Autodesk Inventor part; units mm, degrees
ref_plane "YZ Plane" through (0, 0, 0) normal (1, 0, 0) x (0, 1, 0)
ref_plane "XZ Plane" through (0, 0, 0) normal (0, 1, 0) x (-1, 0, 0)
ref_plane "XY Plane" through (0, 0, 0) normal (0, 0, 1) x (1, 0, 0)
sketch "Sketch1" plane through (0, 0, 0) normal (0, 1, 0) x (-1, 0, 0)
  line L0 (22.5, 10) -> (-22.5, 10)
  line L1 (-22.5, 10) -> (-22.5, -10)
  line L2 (-22.5, -10) -> (22.5, -10)
  line L3 (22.5, -10) -> (22.5, 10)
  line L4 (22.5, 10) -> (-22.5, -10) construction
  line L5 (-22.5, 10) -> (22.5, -10) construction
  point P0 (0, 0)
  dimension "d0" = 45
  dimension "d1" = 20
extrude "Extrusion1" add sketch "Sketch1" along normal blind 5
sketch "Sketch2" plane through (0, 0, 0) normal (0, -1, 0) x (1, 0, 0)
  line L0 (22.5, 10) -> (22.5, -10)
  line L1 (22.5, 10) -> (0, 10)
  line L2 (0, 10) -> (0, 5)
  line L3 (0, 5) -> (22.5, 5)
  line L4 (22.5, 5) -> (22.5, 10)
  point P0 (0, 0)
  dimension "d4" = 22.5
  dimension "d5" = 5
extrude "Extrusion2" add sketch "Sketch2" along normal blind 50
fillet "Fillet1" radius 22.5 1 edges at (0, 0, 7.5)
sketch "Sketch3" plane through (-22.5, 5, 10) normal (0, 0, 1) x (1, 0, 0)
  arc A0 (22.5, -27.5) -> (0, -5) centre (0, -27.5) ccw
  line L0 (22.5, -27.5) -> (22.5, -55)
  line L1 (45, -55) -> (22.5, -55)
  line L2 (45, 0) -> (45, -55)
  line L3 (0, 0) -> (45, 0)
  line L4 (0, -5) -> (0, 0)
  point P0 (22.5, -5)
extrude "Extrusion3" add sketch "Sketch3" along normal blind 15
sketch "Sketch7" plane through (0, 5, 0) normal (0, 1, 0) x (1, 0, 0)
  line L0 (22.5, -5) -> (-22.5, -5)
  line L1 (22.5, 10) -> (22.5, -25)
  line L2 (22.5, -5) -> (22.5, -25)
  line L3 (42.5, -20.5) -> (2.5, -20.5)
  line L4 (2.5, -20.5) -> (2.5, -9.5)
  line L5 (2.5, -9.5) -> (42.5, -9.5)
  line L6 (42.5, -9.5) -> (42.5, -20.5)
  line L7 (42.5, -20.5) -> (2.5, -9.5) construction
  line L8 (2.5, -20.5) -> (42.5, -9.5) construction
  point P0 (0, 0)
  point P1 (22.5, -15)
  dimension "d16" = 40
  dimension "d17" = 11
extrude "Extrusion5" cut sketch "Sketch7" against normal blind 50
sketch "Sketch8" plane through (0, -45, 0) normal (0, 1, 0) x (1, 0, 0)
  line L0 (22.5, -5) -> (22.5, -25)
  line L1 (22.5, -15) -> (7.5, -15)
  line L2 (22.5, -15) -> (37.5, -15) construction
  line L3 (2.5, -20.5) -> (12.5, -20.5)
  line L4 (12.5, -20.5) -> (12.5, -9.5)
  line L5 (12.5, -9.5) -> (2.5, -9.5)
  line L6 (2.5, -9.5) -> (2.5, -20.5)
  line L7 (2.5, -20.5) -> (12.5, -9.5) construction
  line L8 (12.5, -20.5) -> (2.5, -9.5) construction
  line L9 (7.5, -20.5) -> (7.5, -9.5)
  point P0 (0, 0)
  dimension "d20" = 15
  dimension "d21" = 180
  dimension "d22" = 10
  dimension "d23" = 11
extrude "Extrusion6" add sketch "Sketch8" along normal blind 15 contours L9 L3 L6 L5
sketch "Sketch9" plane through (0, -45, 0) normal (0, 1, 0) x (1, 0, 0)
  line L0 (7.5, -9.5) -> (22.5, -9.5)
  line L1 (22.5, -9.5) -> (19.5, -9.5)
  line L2 (19.5, -9.5) -> (19.5, -20.5)
  line L3 (19.5, -20.5) -> (22.5, -20.5)
  line L4 (22.5, -20.5) -> (22.5, -9.5)
  point P0 (0, 0)
  dimension "d26" = 3
  dimension "d27" = 11
extrude "Extrusion7" cut sketch "Sketch9" against normal blind 15
fillet "Fillet2" radius 10 1 edges at (0, -50, 15)
sketch "Sketch10" plane through (-22.5, 5, 25) normal (0, 0, 1) x (1, 0, 0)
  circle A0 centre (32.35, -47.1) radius 1.5
  circle A1 centre (42.65, -24.9) radius 1.5
  point P0 (22.5, -5)
extrude "Extrusion8" cut sketch "Sketch10" against normal blind 20
sketch "Sketch11" plane through (22.5, 0, -10) normal (1, 0, 0) x (0, 0, -1)
  line L0 (-19.5, 5) -> (-19.5, -50)
  line L1 (-15, -50) -> (-19.5, -50)
  line L2 (-15, 0) -> (-15, -50)
  line L3 (-15, 0) -> (0, 0)
  line L4 (0, 0) -> (0, 5)
  line L5 (0, 5) -> (-19.5, 5)
  line L6 (-30.5, -50) -> (-30.5, 5)
  line L7 (-30.5, 5) -> (-35, 5)
  line L8 (-35, -50) -> (-35, 5)
  line L9 (-30.5, -50) -> (-35, -50)
  point P0 (-10, 0)
extrude "Extrusion9" add sketch "Sketch11" along normal blind 5
sketch "Sketch12" plane through (0, -50, 0) normal (0, -1, 0) x (1, 0, 0)
  line L0 (10, 5) -> (27.5, 5)
  line L1 (27.5, 5) -> (22.5, 5)
  line L2 (22.5, 5) -> (22.5, 25)
  line L3 (22.5, 25) -> (27.5, 25)
  line L4 (27.5, 25) -> (27.5, 5)
  point P0 (0, 0)
  dimension "d35" = 5
  dimension "d36" = 20
extrude "Extrusion10" cut sketch "Sketch12" against normal blind 25
fillet "Fillet3" radius 10 4 edges at (27.5, -25, 7.25) (22.5, -25, 7.25) (27.5, -25, 22.75) (22.5, -25, 22.75)
sketch "Sketch13" plane through (0, 0, 0) normal (0, -1, 0) x (1, 0, 0)
  line L0 (27.5, -10) -> (17.5, -10)
  line L1 (17.5, -10) -> (17.5, 5)
  line L2 (17.5, 5) -> (27.5, 5)
  line L3 (27.5, 5) -> (27.5, -10)
  point P0 (0, 0)
  dimension "d40" = 10
  dimension "d41" = 15
extrude "Extrusion11" add sketch "Sketch13" along normal blind 10
sketch "Sketch14" plane through (0, 5, 0) normal (0, 1, 0) x (1, 0, 0)
  line L0 (-22.5, 10) -> (27.5, 10)
  line L1 (-22.5, 10) -> (-13, 10)
  line L2 (-13, 10) -> (-13, 5)
  line L3 (-13, 5) -> (3, 5)
  circle A0 centre (-13, 5) radius 2.5
  circle A1 centre (3, 5) radius 2.5
  point P0 (0, 0)
  dimension "d45" = 9.5
  dimension "d46" = 5
  dimension "d47" = 16
  dimension "d48" = 90
  dimension "d49" = 5
  dimension "d50" = 5
extrude "Extrusion12" cut sketch "Sketch14" against normal blind 10
sketch "Sketch15" plane through (-22.5, 0, -10) normal (0, 0, -1) x (-1, 0, 0)
  line L0 (0, 0) -> (-40, 0)
  line L1 (0, 0) -> (0, 5)
  line L2 (0, 5) -> (-50, 5)
  line L3 (-50, 5) -> (-50, -10)
  line L4 (-40, -10) -> (-50, -10)
  line L5 (-40, 0) -> (-40, -10)
  point P0 (-22.5, 0)
extrude "Extrusion13" add sketch "Sketch15" along normal blind 5
fillet "Fillet5" radius 5 1 edges at (-2.5, 0, -15)
fillet "Fillet6" radius 5 2 edges at (22.5, -10, 5) (22.5, -10, -15)
fillet "Fillet7" radius 22 1 edges at (27.5, 5, 22.75)
fillet "Fillet8" radius 5 1 edges at (27.5, 5, -2.75)
properties part number "SOPORTE_FDC"
Work out the finished part from the listing and answer in its coordinate system (mm). A direction names the side the tool comes from. Give positions to 0.01 mm unless a question says otherwise; leave off trailing zeros. Loops run counter-clockwise (first coordinate to the right, second up) from the corner with the lowest first, then second, coordinate; pieces in that order, holes last. Notation, with made-up numbers: M -28,41.5 L -11,41.5 A13 cw -11,50.5 Z; hole C 66.5,20 d9. An arc over 180 degrees is marked long. One line per item, written item: value. Start each with the question number.
1. Find the intervals of material crossed by probe 1 along Z at (x, y) = (9.5, -27.5); probe 2 along X at (y, z) = (1.55, -5); probe 3 along Y at (x, z) = (9.85, 6.45), in increasing order.
2. Find section D-D (y = -42.1). Give the vertices of the cut face in (x, z).
3. Find section B-B (z = 8). State how many separate pieces and enclosed holes the cut face has, and give its area (3 significant figures).
4. Find section A-A (z = -5). Give the vertices of the cut face in (x, y).
5. Each of these flat-tipped pins is pushed along its axis until it touches: P1, Ø4.5, axis at x = -13, z = -5, coming from the -Y side; P2, Ø4, axis at y = -46.5, z = 16.5, coming from the +X side; P3, Ø4, axis at x = 20.15, y = -19.9, coming from the -Z side; P4, Ø3, axis at y = -5.5, z = 20.5, coming from the -X side. Where does it stop, or does it pass through?
6. Which of the six approach directions +Z, -Z, +X, -X, +Y, -Y give full straight-line access (tool end or side, diameter ignored) to faces 4 (the face through (19.5, -47, 15)), 5 (the face through (15, -16, 9.5)), 6 (the face through (-3, 0, -2))?
7. Determine the mould class of faces 1 (the face through (27.5, -8, 0)), 2 (the face through (8, -25, 5)), 3 (the face through (7.5, -38, 15)) for opening direction Z: released by +Z, released by -Z, zero draft, split by the parting line, or undercut.
Reported:
1. probe 1: z = 5 to 9.5, 20.5 to 25
1. probe 2: x = -22.5 to -15.5, -10.5 to 0.5, 5.5 to 27.25
1. probe 3: y = -50 to -43.6, -40.6 to 5
2. outline: M 0.22,5 L 8.35,5 L 8.35,9.5 L 7.5,9.5 L 7.5,20.5 L 8.35,20.5 L 8.35,25 L 0.22,25 Z; M 11.35,5 L 22.5,5 L 22.5,9.5 L 11.35,9.5 Z; M 11.35,20.5 L 22.5,20.5 L 22.5,25 L 11.35,25 Z
3. separate pieces: 1
3. enclosed holes: 2
3. area: 1,580 mm²
4. outline: M -22.5,0 L -15.5,0 L -15.5,5 L -22.5,5 Z; M -10.5,0 L 0.5,0 L 0.5,5 L -10.5,5 Z; M 5.5,0 L 17.5,0 L 17.5,-10 L 27.5,-10 L 27.5,0 A5 ccw 22.5,5 L 5.5,5 Z
5. P1: passes through
5. P2: stops at x = 19.5
5. P3: stops at z = 5
5. P4: stops at x = -9.69
6. face 4: +X, +Y, -Y
6. face 5: +X, +Y
6. face 6: -Z, -X, -Y
7. face 1: zero draft
7. face 2: released by -Z
7. face 3: undercut
